```python
from build123d import *

# Parameters (mm, degrees)
SKETCH010_R                               = 1.25
EXTRUDE009_DEPTH                          = 1.5
SKETCH009_R                               = 2
SKETCH009_R_2                             = 15
EXTRUDE008_DEPTH                          = 1.5
SKETCH008_R                               = 1.5
EXTRUDE007_DEPTH                          = 1.5
EXTRUDE006_DEPTH                          = 1.5
EXTRUDE006_ONTO_SKETCH007_PLACEMENT_ANGLE = 90.001496
FILLET_R                                  = 2.5


with BuildPart() as obj1:
    # Sketch010 (on Face2 of Cut002) → Extrude009 (new body)
    with BuildSketch(Plane(origin=(0, 0, 39.25), x_dir=(1, 0, 0), z_dir=(0, 0, -1))):
        with Locations((-18, -23.5)):
            Circle(SKETCH010_R)
        with Locations((18, -23.5)):
            Circle(SKETCH010_R)
        with Locations((18, 23.5)):
            Circle(SKETCH010_R)
        with Locations((-18, 23.5)):
            Circle(SKETCH010_R)
        with Locations((23.5, -18)):
            Circle(SKETCH010_R)
        with Locations((23.5, 18)):
            Circle(SKETCH010_R)
        with Locations((-23.5, -18)):
            Circle(SKETCH010_R)
        with Locations((-23.5, 18)):
            Circle(SKETCH010_R)
    extrude(amount=EXTRUDE009_DEPTH)


with BuildPart() as obj1_1:
    # Extrude009 placement: moved
    add(obj1.part.moved(Location((0, 0, -38.5))))


with BuildPart() as pcb_mount_holes_bot:
    # Sketch009 (on Face4 of Cut001) → Extrude008 (new body)
    with BuildSketch(Plane.XY.offset(41)):
        with Locations((0, -30)):
            Circle(SKETCH009_R)
        with Locations((-30, 0)):
            Circle(SKETCH009_R)
        with Locations((0, 30)):
            Circle(SKETCH009_R)
        with Locations((30, 0)):
            Circle(SKETCH009_R)
        Circle(SKETCH009_R_2)
    extrude(amount=EXTRUDE008_DEPTH)


with BuildPart() as pcb_mount_holes_bot_1:
    # Extrude008 placement: moved
    add(pcb_mount_holes_bot.part.moved(Location((0, 0, -41.75))))


with BuildPart() as new_bottom_plate_holes:
    # Sketch008 (on Face10 of Extrude006) → Extrude007 (new body)
    with BuildSketch(Plane.XY.offset(0.75)):
        with Locations((31.5, -46.3)):
            Circle(SKETCH008_R)
        with Locations((-31.5, -46.3)):
            Circle(SKETCH008_R)
        with Locations((46.3, -31.5)):
            Circle(SKETCH008_R)
        with Locations((-46.3, -31.5)):
            Circle(SKETCH008_R)
        with Locations((46.3, 31.5)):
            Circle(SKETCH008_R)
        with Locations((-46.3, 31.5)):
            Circle(SKETCH008_R)
        with Locations((-31.5, 46.3)):
            Circle(SKETCH008_R)
        with Locations((31.5, 46.3)):
            Circle(SKETCH008_R)
    extrude(amount=EXTRUDE007_DEPTH)


with BuildPart() as new_bottom_plate_holes_1:
    # Extrude007 placement: moved
    add(new_bottom_plate_holes.part.moved(Location((0, 0, -1.5))))


with BuildPart() as bottom_plate_new:
    # Sketch007 as drawn → Extrude006 (new)
    with BuildSketch(Plane.XY):
        with BuildLine():
            Line((-54.41461, 31.12), (-31.098088, 54.458425))
            ThreePointArc((-31.098088, 54.458425), (-0.589258, 41.589673), (30.25328, 53.63672))
            Line((52.777302, 31.112698), (30.25328, 53.63672))
            ThreePointArc((52.777302, 31.112698), (39.890076, -0.081699), (52.893056, -31.228024))
            Line((31.098088, -53.043466), (52.893056, -31.228024))
            ThreePointArc((31.098088, -53.043466), (-0.487382, -40.173467), (-31.78, -53.74))
            Line((-31.78, -53.74), (-54.4, -31.12))
            ThreePointArc((-54.4, -31.12), (-41.5127, 0.003027), (-54.41461, 31.12))
        make_face()
    extrude(amount=EXTRUDE006_DEPTH)


with BuildPart() as bottom_plate_new_1:
    # Extrude006 onto Sketch007 placement: moved
    add(bottom_plate_new.part.moved(Location((-0.000606, 0.67074, -0.75))).rotate(Axis((-0.000606, 0.67074, -0.75), (0, 0, 1)), EXTRUDE006_ONTO_SKETCH007_PLACEMENT_ANGLE))

    # Cut005: cut new_bottom_plate_holes
    add(new_bottom_plate_holes_1.part, mode=Mode.SUBTRACT)

    # Cut006: cut pcb_mount_holes_bot
    add(pcb_mount_holes_bot_1.part, mode=Mode.SUBTRACT)

    # Cut007: cut obj1
    add(obj1_1.part, mode=Mode.SUBTRACT)

    # Fillet
    fillet_edges = [bottom_plate_new_1.edges().sort_by_distance(p)[0] for p in [
        (53.042048, 31.770213, 0),
        (53.740224, -31.107857, 0),
        (31.226037, 53.564611, 0),
        (31.120814, -53.728448, 0),
        (-31.114682, 53.447229, 0),
        (-31.119185, -53.744683, 0),
        (-53.638116, 30.92262, 0),
        (-54.458219, -30.42877, 0),
    ]]
    fillet(fillet_edges, radius=FILLET_R)


solid = bottom_plate_new_1.part
```
Work out the finished part from the listing and answer in its coordinate system (mm). Give positions to 0.01 mm unless a question says otherwise; leave off trailing zeros. Order: outer loops, then holes, each group sorted by start corner. A loop starts at its lowest first (then second) coordinate and runs counter-clockwise, first axis right, second up. Notation, with made-up numbers: (-16.75, 44) - (9.25, 44) arc R34 ccw to (9.25, 78) - close; hole circle Ø8 at (21.5, -16). An arc over 180 degrees is marked (long way). One line per item, written item: value. Start each with the question number.
1. Section C-C, the plane y = 10.5 is taken. Write down the section's boundary in (x, z), then the cut area to 3 significant figures.
2. Consider line 1 (Y direction, x = 23.5, z = -0.2); line 2 (Y direction, x = 18, z = -0.2); line 3 (Y direction, x = -31.5, z = 0.35). Determine where each line is inside the solid, lowest interval first.
3. Section D-D, the plane y = -46.3 is taken. Write down the section's boundary in (x, z), then the cut area to 3 significant figures.
4. Section B-B, the plane y = -18 is taken. Write down the section's boundary in (x, z).
5. Section A-A, the plane x = 0 is taken. Write down the section's boundary in (y, z), then the cut area to 3 significant figures.
6. For a pull along X with two mould halves and no side action, classify faces 1 (the face through (40.17, 0.67, -0.01)), 2 (the face through (-22.31, 17.62, 0.01)), 3 (the face through (11, -11, -0.75)) as released by +X, released by -X, zero draft, split by the parting line, or undercut.
Filled sheet:
1. outline: (-42.7, -0.75) - (-10.71, -0.75) - (-10.71, 0.75) - (-42.7, 0.75) - close; (10.71, -0.75) - (41.28, -0.75) - (41.28, 0.75) - (10.71, 0.75) - close
1. area: 93.8 mm²
2. line 1: -47.64 to -19.25, -16.75 to 16.75, 19.25 to 47.36
2. line 2: -44.69 to -24.75, -22.25 to 22.25, 24.75 to 44.41
2. line 3: -52.72 to -47.8, -44.8 to -1.32, 1.32 to 44.8, 47.8 to 52.42
3. outline: (-38.57, -0.75) - (-33, -0.75) - (-33, 0.75) - (-38.57, 0.75) - close; (-30, -0.75) - (-21.22, -0.75) - (-21.22, 0.75) - (-30, 0.75) - close; (21.23, -0.75) - (30, -0.75) - (30, 0.75) - (21.23, 0.75) - close; (33, -0.75) - (38.55, -0.75) - (38.55, 0.75) - (33, 0.75) - close
3. area: 43.0 mm²
4. outline: (-45.74, -0.75) - (-24.75, -0.75) - (-24.75, 0.75) - (-45.74, 0.75) - close; (-22.25, -0.75) - (22.25, -0.75) - (22.25, 0.75) - (-22.25, 0.75) - close; (24.75, -0.75) - (44.33, -0.75) - (44.33, 0.75) - (24.75, 0.75) - close
5. outline: (-40.84, -0.75) - (-32, -0.75) - (-32, 0.75) - (-40.84, 0.75) - close; (-28, -0.75) - (-15, -0.75) - (-15, 0.75) - (-28, 0.75) - close; (15, -0.75) - (28, -0.75) - (28, 0.75) - (15, 0.75) - close; (32, -0.75) - (40.56, -0.75) - (40.56, 0.75) - (32, 0.75) - close
5. area: 65.1 mm²
6. face 1: released by +X
6. face 2: undercut
6. face 3: zero draft
